Input: dimensioned drawing with shaded views. Units: mm. Origin: part minimum x, y, z. A direction names the side the tool comes from. Round coordinates to 2 decimals unless told otherwise and drop trailing zeros. Order: outer loops, then holes, each group sorted by start corner. A loop starts at its lowest first (then second) coordinate and runs counter-clockwise, first axis right, second up.
Item 1: Line query: L1, parallel to Z at x = 15.5, y = 4.7; L2, parallel to Z at x = 7.25, y = 4.3; L3, parallel to X at y = 3.5, z = 15. Output: solid intervals per line, ascending.
Item 2: Mould query, pull axis Z, two halves, no side actions, for the marked faces 3, 4 and 5. Classes: released by +Z, released by -Z, zero draft, split by the parting line, or undercut.
Item 3: Cut plane A-A on z = 4. Output: boundary loops of the cut face in (x, y), then the cut area to 3 significant figures.
Item 4: Reachability of the marked faces 1 and 2 from +Z, -Z, +X, -X, +Y, -Y: full face, straight path, thin tool, end or side. Return the list, or none.
Item 5: First-contact query: pin 1 (1.5 mm diameter, centred on x = 2, y = 3, fed in from +Z); pin 2 (3 mm diameter, centred on x = 13, y = 3, fed in from -Z); pin 3 (1.1 mm diameter, centred on x = 15, y = 3, fed in from +Z). Flat tips, straight axial feed; report the tip coordinate or a pass-through.
Item 6: Cut plane D-D on x = 18.25. Output: boundary loops of the cut face in (y, z).
Item 7: Cut plane B-B on x = 7. Output: boundary loops of the cut face in (y, z).
Item 8: Cut plane C-C on y = 3.2. Output: boundary loops of the cut face in (x, z), then the cut area to 3 significant figures.
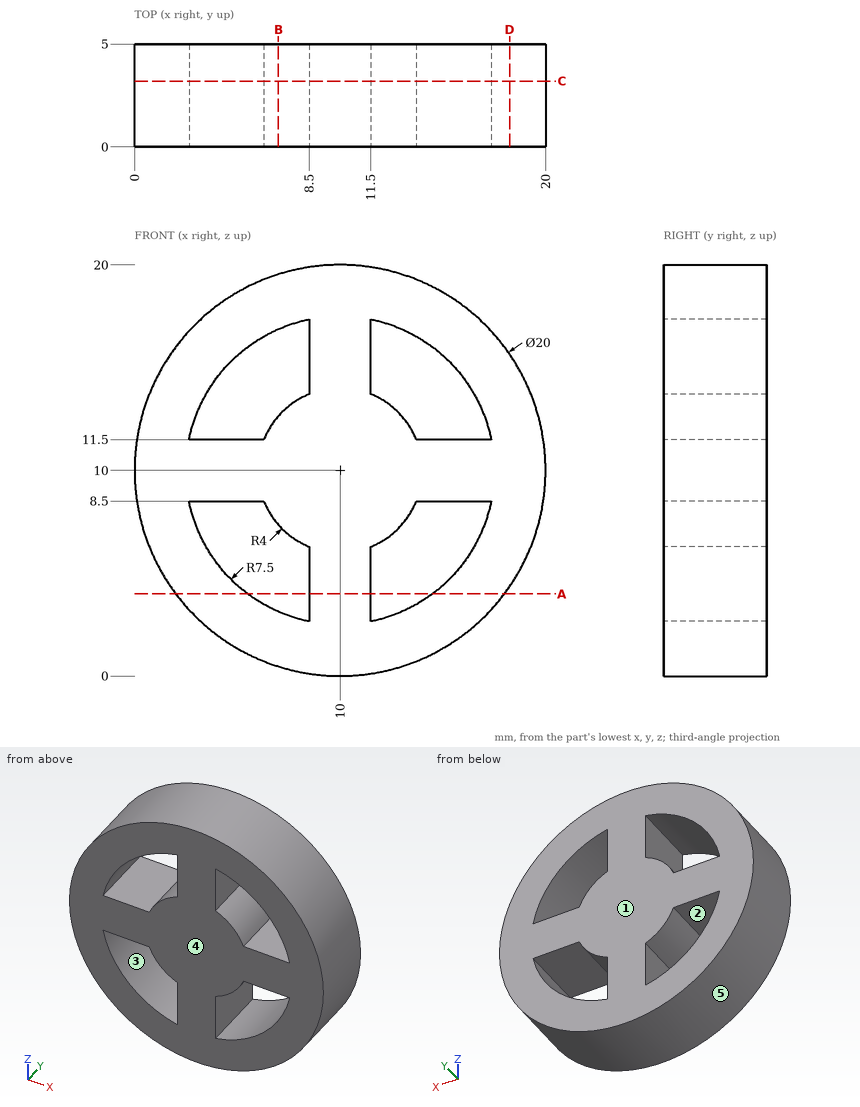
From the geometry:
1. L1: z = 1.65 to 4.9, 8.5 to 11.5, 15.1 to 18.35
1. L2: z = 0.39 to 3.02, 7.1 to 12.9, 16.98 to 19.61
1. L3: x = 1.34 to 4.41, 8.5 to 11.5, 15.59 to 18.66
2. face 3: undercut
2. face 4: zero draft
2. face 5: split by the parting line
3. outline: (2, 0) - (5.5, 0) - (5.5, 5) - (2, 5) - close; (8.5, 0) - (11.5, 0) - (11.5, 5) - (8.5, 5) - close; (14.5, 0) - (18, 0) - (18, 5) - (14.5, 5) - close
3. area: 50.0 mm2
4. face 1: +Z, -Z, +X, -X, +Y
4. face 2: +Y, -Y
5. pin 1: stops at z = 16.89
5. pin 2: stops at z = 0.11
5. pin 3: stops at z = 18.96
6. outline: (0, 4.35) - (5, 4.35) - (5, 15.65) - (0, 15.65) - close
7. outline: (0, 0.46) - (5, 0.46) - (5, 3.13) - (0, 3.13) - close; (0, 7.35) - (5, 7.35) - (5, 12.65) - (0, 12.65) - close; (0, 16.87) - (5, 16.87) - (5, 19.54) - (0, 19.54) - close
8. outline: circle Ø20 at (10, 10); hole (2.65, 8.5) arc R7.5 ccw to (8.5, 2.65) - (8.5, 6.29) arc R4 cw to (6.29, 8.5) - close; hole (2.65, 11.5) - (6.29, 11.5) arc R4 cw to (8.5, 13.71) - (8.5, 17.35) arc R7.5 ccw to start; hole (11.5, 2.65) arc R7.5 ccw to (17.35, 8.5) - (13.71, 8.5) arc R4 cw to (11.5, 6.29) - close; hole (11.5, 13.71) arc R4 cw to (13.71, 11.5) - (17.35, 11.5) arc R7.5 ccw to (11.5, 17.35) - close
8. area: 230 mm2
